Can you work these out from the model? Positions are in its coordinate system, mm. A direction names the side the tool comes from. Round coordinates to 2 decimals unless told otherwise and drop trailing zeros. Write each loop counter-clockwise with the first axis right and the second up, starting at its lowest first coordinate (ties: lowest second). Pieces come first, ordered by that corner, then holes. Notation, with made-up numbers: M -14,88 L 8,88 A19 ccw 8,92 Z; hole C -25.75,71.25 d4. An arc over 180 degrees is marked long. Answer as a JSON object with one key per item and string values. Group by question number.
1) Suppose I cut it at B-B, the plane x = 142.5. Write out the boundary of the cut face in (y, z).
2) If we mould it in two halves opening along X, with no side actions, what happens to faces 4 (the flat face through (44.196, 112, -50)), 5 (the flat face through (3, 49, -101.6)), 6 (the flat face through (88, 90, 6.35))? For each: +X half, -X half, draft (parallel to the pull), parting line (faces both ways), or undercut.
3) Please list where these lines run through material, in increasing order: L1, parallel to X at y = 122.5, z = -22; L2, parallel to X at y = 10, z = 13.5. Write a range as [from, to].
4) On a 3-axis mill with a long thin cutter (end or side, diameter ignored), from which of +Z, -Z, +X, -X, +Y, -Y can I reach the whole of each face in a straight line? I mean faces 1 (the flat face through (171.45, 88, 16)), 2 (the flat face through (110, 112, 0)), 3 (the flat face through (109, 37.846, -50)). Say none if no direction works.
5) I'm going to push flat-ended pins straight in: pin 1 Ø1.5 at (y, z) = (121, -36) entering from +X; pin 2 Ø4 at (x, y) = (22.5, 52.5) entering from -Z; pin 3 Ø3 at (x, z) = (33, -77.5) entering from +Y. Where does each tip first touch, or does it pass through?
6) Suppose I cut it at A-A, the plane z = -20. Write out the boundary of the cut face in (x, y), and give its area (3 significant figures).
from build123d import *

# Parameters (mm, degrees)
F0_W     = 177.8
F0_H     = 177.8
F0_W_2   = 165.1
F0_H_2   = 165.1
F1_DEPTH = 25.4
F2_DEPTH = 6.35
F4_DEPTH = 101.6
F6_DEPTH = 101.6


with BuildPart() as f1:
    # F0 (on Top) → F1 (new body)
    with BuildSketch(Plane.XY):
        with Locations((88.9, 88.9)):
            Rectangle(F0_W, F0_H)
        with Locations((88.9, 88.9)):
            Rectangle(F0_W_2, F0_H_2, mode=Mode.SUBTRACT)
    extrude(amount=F1_DEPTH)

    # F0 (on Top) → F2 (join)
    with BuildSketch(Plane.XY):
        with Locations((88.9, 88.9)):
            Rectangle(F0_W_2, F0_H_2)
    extrude(amount=F2_DEPTH)

    # F3 (on face) → F4 (join)
    with BuildSketch(Plane(origin=(0, 0, 0), x_dir=(1, 0, 0), z_dir=(0, 0, -1))):
        Polygon((177.8, 0), (0, 0), (0, -177.8), (6.35, -177.8), (6.35, -6.35), (177.8, -6.35), align=None)
    extrude(amount=F4_DEPTH)

    # F5 (on face) → F6 (join)
    with BuildSketch(Plane(origin=(0, 0, 0), x_dir=(1, 0, 0), z_dir=(0, 0, -1))):
        Polygon((37.846, -37.846), (37.846, -177.8), (44.196, -177.8), (44.196, -44.196), (177.8, -44.196), (177.8, -37.846), align=None)
    extrude(amount=F6_DEPTH)


solid = f1.part
Results:
{
 "1": {"outline": "M 0,-101.6 L 6.35,-101.6 L 6.35,0 L 37.85,0 L 37.85,-101.6 L 44.2,-101.6 L 44.2,0 L 177.8,0 L 177.8,25.4 L 171.45,25.4 L 171.45,6.35 L 6.35,6.35 L 6.35,25.4 L 0,25.4 Z"},
 "2": {"face 4": "+X half", "face 5": "draft", "face 6": "undercut"},
 "3": {"L1": "[0, 6.35], [37.85, 44.2]", "L2": "[0, 6.35], [171.45, 177.8]"},
 "4": {"face 1": "+Z", "face 2": "-Z, +X, +Y", "face 3": "-Z, +X"},
 "5": {"pin 1": "x = 44.2", "pin 2": "z = 0", "pin 3": "y = 6.35"},
 "6": {"outline": "M 0,0 L 177.8,0 L 177.8,6.35 L 6.35,6.35 L 6.35,177.8 L 0,177.8 Z; M 37.85,37.85 L 177.8,37.85 L 177.8,44.2 L 44.2,44.2 L 44.2,177.8 L 37.85,177.8 Z", "area": "3,950 mm^2"}
}
